Build history of the part. All positions in model axes, mm. A direction names the side the tool comes from. Coordinates: 2 decimals unless noted, no trailing zeros. Loops run counter-clockwise (first coordinate to the right, second up) from the corner with the lowest first, then second, coordinate; pieces in that order, holes last. Notation, with made-up numbers: (77, -11) -> (123, -11) arc R16 ccw to (123, -5) -> close; hole circle Ø1 at (58, 85.25). An arc over 180 degrees is marked (long way). One line per item, written item: value. Start each with the question number.
Autodesk Inventor part; units mm, degrees
ref_plane "Work Plane1" through (0, 14, 0) normal (0, -1, 0) x (1, 0, 0)
ref_plane "YZ Plane" through (0, 0, 0) normal (1, 0, 0) x (0, 1, 0)
ref_plane "XZ Plane" through (0, 0, 0) normal (0, 1, 0) x (-1, 0, 0)
sketch "Sketch1" plane through (0, 0, 0) normal (0, 1, 0) x (-1, 0, 0)
  circle A0 centre (0, 0) radius 9.8
  dimension "d0" = 19.6
extrude "Extrusion1" add sketch "Sketch1" along normal blind 20
ref_plane "Work Plane1" through (0, 14, 0) normal (0, -1, 0) x (1, 0, 0)
sketch "Sketch3" plane through (0, 14, 0) normal (0, -1, 0) x (1, 0, 0)
  circle A0 centre (0, 0) radius 12.5
  dimension "d7" = 25
extrude "Extrusion3" add sketch "Sketch3" against normal blind 3
shell "Shell1" thickness 2.5 removed faces 2 at (0.3035, 20, 2.5) at (0.3035, 0, 2.5)
properties part number "Pomodoro Robot Neck"
Item 1: Probe probe 1 along X at (y, z) = (7.5, 0); probe 2 along Z at (x, y) = (-4.25, 13.5). List the from-to ranges inside material, lowest first.
Item 2: Band-saw the part on A-A, the plane x = 0. List the corners of the cut face in (y, z).
Item 3: Drop flat-ended pins along their axis: pin 1 Ø4 at (y, z) = (7.5, -8) entering from -X; pin 2 Ø9 at (x, z) = (0, 0) entering from -Y; pin 3 Ø6 at (x, y) = (8.5, 5) entering from +Z; pin 4 Ø2 at (x, z) = (-9.5, 7) entering from -Y. Give the stop position or say it passes through.
Item 4: Band-saw the part on D-D, the plane z = -9. List the corners of the cut face in (x, y), and give its area (3 significant figures).
Item 5: Tool access for faces 1 (the face through (2.124, 18.479, 9.567)), 2 (the face through (5.5, 14, -8.3)), 3 (the face through (1.5, 20, 7.3)): list every direction of +Z, -Z, +X, -X, +Y, -Y with a clear straight run to the whole face (end or side of a thin tool).
Item 6: Band-saw the part on B-B, the plane z = -2. List the corners of the cut face in (x, y), and give its area (3 significant figures).
Item 7: Band-saw the part on C-C, the plane y = 5.5. List the corners of the cut face in (x, z).
Worked out:
1. probe 1: x = -9.8 to -7.3, 7.3 to 9.8
1. probe 2: z = -8.83 to -5.94, 5.94 to 8.83
2. outline: (0, -9.8) -> (14, -9.8) -> (14, -12.5) -> (17, -12.5) -> (17, -9.8) -> (20, -9.8) -> (20, -7.3) -> (14, -7.3) -> (0, -7.3) -> close; (0, 7.3) -> (20, 7.3) -> (20, 9.8) -> (17, 9.8) -> (17, 12.5) -> (14, 12.5) -> (14, 9.8) -> (0, 9.8) -> close
3. pin 1: stops at x = -7.75
3. pin 2: passes through
3. pin 3: stops at z = 8.11
3. pin 4: stops at y = 14
4. outline: (-8.67, 14) -> (-3.88, 14) -> (-3.88, 0) -> (3.88, 0) -> (3.88, 14) -> (8.67, 14) -> (8.67, 17) -> (3.88, 17) -> (3.88, 20) -> (-3.88, 20) -> (-3.88, 17) -> (-8.67, 17) -> close
4. area: 184 mm²
5. face 1: +Y
5. face 2: -Y
5. face 3: +Z, -Z, +X, -X, +Y
6. outline: (-12.34, 14) -> (-9.59, 14) -> (-9.59, 0) -> (-7.02, 0) -> (-7.02, 20) -> (-9.59, 20) -> (-9.59, 17) -> (-12.34, 17) -> close; (7.02, 0) -> (9.59, 0) -> (9.59, 14) -> (12.34, 14) -> (12.34, 17) -> (9.59, 17) -> (9.59, 20) -> (7.02, 20) -> (7.02, 14) -> close
6. area: 119 mm²
7. outline: circle Ø19.6 at (0, 0); hole circle Ø14.6 at (0, 0)
